Design review of the part shown in the three views and the two pictorial views. Dimensions are in mm from the part's minimum x, y and z. A direction names the side the tool comes from. Round coordinates to 2 decimals unless told otherwise and drop trailing zeros. Loops run counter-clockwise (first coordinate to the right, second up) from the corner with the lowest first, then second, coordinate; pieces in that order, holes last.
1. Consider section C-C on x = 17.3. State the section outline as (y, z) points, then the cut area to 3 significant figures.
2. Consider section D-D on z = 17.3. State the section outline as (x, y) points.
3. To check wall thickness, follow line 1 along X through (y, z) = (2, 17.3); line 2 along Z through (x, y) = (17.3, 3.75); line 3 along X through (y, z) = (5.5, 18). State the ranges of each line that lie inside material, in increasing order.
4. Tool access review of the marked faces 4, 5, 6 and 7: name each direction out of +Z, -Z, +X, -X, +Y, -Y from which nothing blocks a thin tool from reaching the whole face with its end or side.
5. Consider section B-B on y = 3.25. State the section outline as (x, z) points, then the cut area to 3 significant figures.
6. Draft analysis for pull direction X (two halves, no side actions). For the marked faces 1, 2 and 3, state which applies: released by +X, released by -X, zero draft, split by the parting line, or undercut.
7. Consider section A-A on z = 31.45. State the section outline as (x, y) points, then the cut area to 3 significant figures.
8. Clearance check with flat-ended pins moving along their axes: pin 1 Ø2.5 at (x, y) = (31, 3) entering from +Z; pin 2 Ø0.7 at (x, y) = (31, 4.5) entering from -Z; pin 3 Ø1.5 at (x, y) = (9.5, 2) entering from -Z. State where each tip first meets the part, or that it passes through.
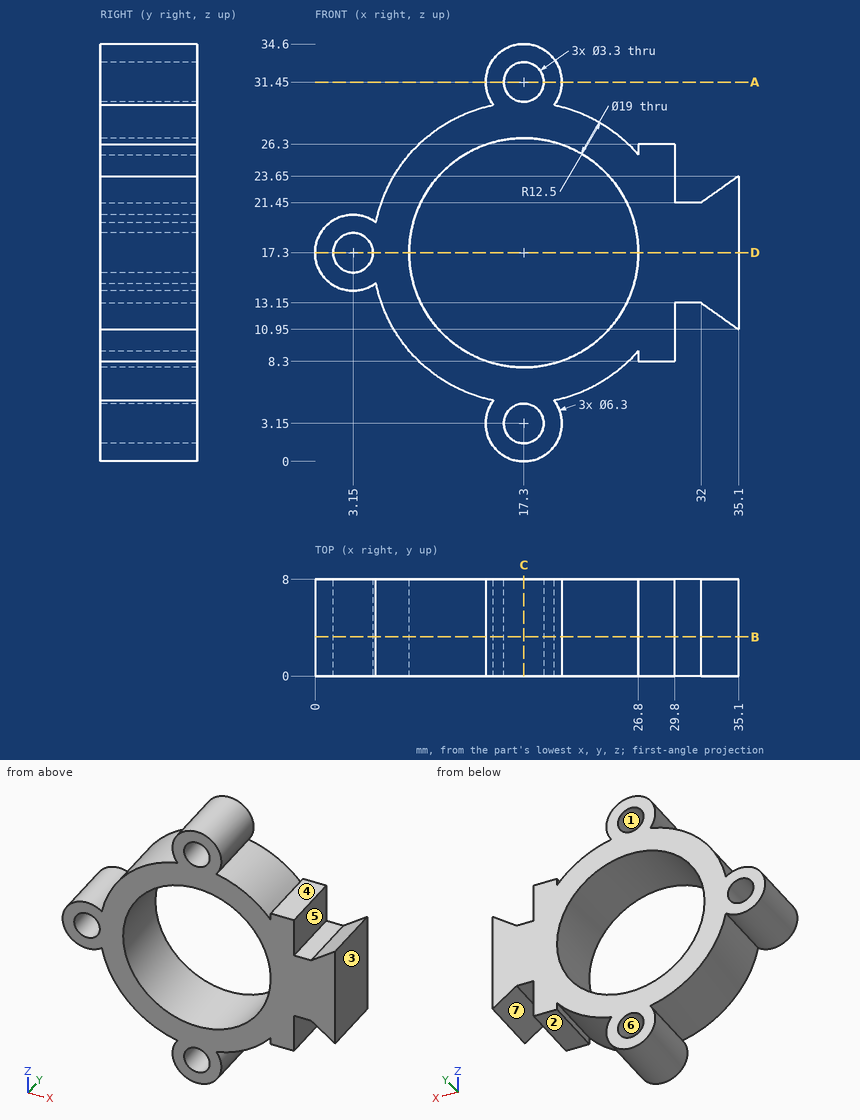
Resolved:
1. outline: (0, 0) - (8, 0) - (8, 1.5) - (0, 1.5) - close; (0, 4.8) - (8, 4.8) - (8, 7.8) - (0, 7.8) - close; (0, 26.8) - (8, 26.8) - (8, 29.8) - (0, 29.8) - close; (0, 33.1) - (8, 33.1) - (8, 34.6) - (0, 34.6) - close
1. area: 72.0 mm2
2. outline: (0, 0) - (1.5, 0) - (1.5, 8) - (0, 8) - close; (4.8, 0) - (7.8, 0) - (7.8, 8) - (4.8, 8) - close; (26.8, 0) - (35.1, 0) - (35.1, 8) - (26.8, 8) - close
3. line 1: x = 0 to 1.5, 4.8 to 7.8, 26.8 to 35.1
3. line 2: z = 0 to 1.5, 4.8 to 7.8, 26.8 to 29.8, 33.1 to 34.6
3. line 3: x = 0.08 to 1.66, 4.64 to 7.83, 26.77 to 35.1
4. face 4: +Z, +X, +Y, -Y
4. face 5: +Z, +Y, -Y
4. face 6: +Y, -Y
4. face 7: -Z, +Y, -Y
5. outline: (5.05, 14.79) arc R12.5 ccw to (14.79, 5.05) arc R3.15 ccw (long way) to (19.81, 5.05) arc R12.5 ccw to (26.8, 9.18) - (26.8, 8.3) - (29.8, 8.3) - (29.8, 13.15) - (32, 13.15) - (35.1, 10.95) - (35.1, 23.65) - (32, 21.45) - (29.8, 21.45) - (29.8, 26.3) - (26.8, 26.3) - (26.8, 25.42) arc R12.5 ccw to (19.81, 29.55) arc R3.15 ccw (long way) to (14.79, 29.55) arc R12.5 ccw to (5.05, 19.81) arc R3.15 ccw (long way) to start; hole circle Ø3.3 at (3.15, 17.3); hole circle Ø19 at (17.3, 17.3); hole circle Ø3.3 at (17.3, 3.15); hole circle Ø3.3 at (17.3, 31.45)
5. area: 331 mm2
6. face 1: undercut
6. face 2: zero draft
6. face 3: released by +X
7. outline: (14.15, 0) - (15.65, 0) - (15.65, 8) - (14.15, 8) - close; (18.95, 0) - (20.45, 0) - (20.45, 8) - (18.95, 8) - close
7. area: 24.0 mm2
8. pin 1: stops at z = 26.3
8. pin 2: stops at z = 13.15
8. pin 3: stops at z = 6.98
